The figure shows three views and two pictorial views of one solid part (mm, origin at its lowest corner). Answer the questions. Round coordinates to 2 decimals unless told otherwise and drop trailing zeros. Order: outer loops, then holes, each group sorted by start corner. A loop starts at its lowest first (then second) coordinate and runs counter-clockwise, first axis right, second up. Notation, with made-up numbers: (68.5, 39.25) - (116.5, 39.25) arc R32 cw to (116.5, 71.25) - close; hole circle Ø7 at (31.25, -17). An arc over 180 degrees is marked (long way). Answer as a JSON object with one key per item and string values. Group by question number.
Q1. A cutting plane is placed at A-A on x = 58.5. Determine the outline of the cut face in (y, z).
Q2. Consider line 1 (Z direction, x = 58.5, y = 3.1); line 2 (Z direction, x = 8, y = 2.4); line 3 (X direction, y = 4.3, z = 69) (1 decimal). Determine where each line is inside the solid, lowest interval first.
Q3. A cutting plane is placed at D-D on z = 24. Determine the outline of the cut face in (x, y), and give its area (3 significant figures).
Q4. A cutting plane is placed at C-C on y = 0.75. Count the separate pieces of the cut face and the enclosed holes in it, and give its area (3 significant figures).
Q5. A cutting plane is placed at B-B on z = 7.5. Determine the outline of the cut face in (x, y).
Q6. Given pin 1 Ø5.5 at (x, z) = (9.99, 69.75) entering from +Y; pin 2 Ø4.5 at (x, z) = (9.99, 29.75) entering from -Y (1 decimal); pin 3 Ø1 at (y, z) = (1.5, 74.5) entering from +X, each flat-ended and moving along its own axis, determine where each tip first touches the part or whether it passes through.
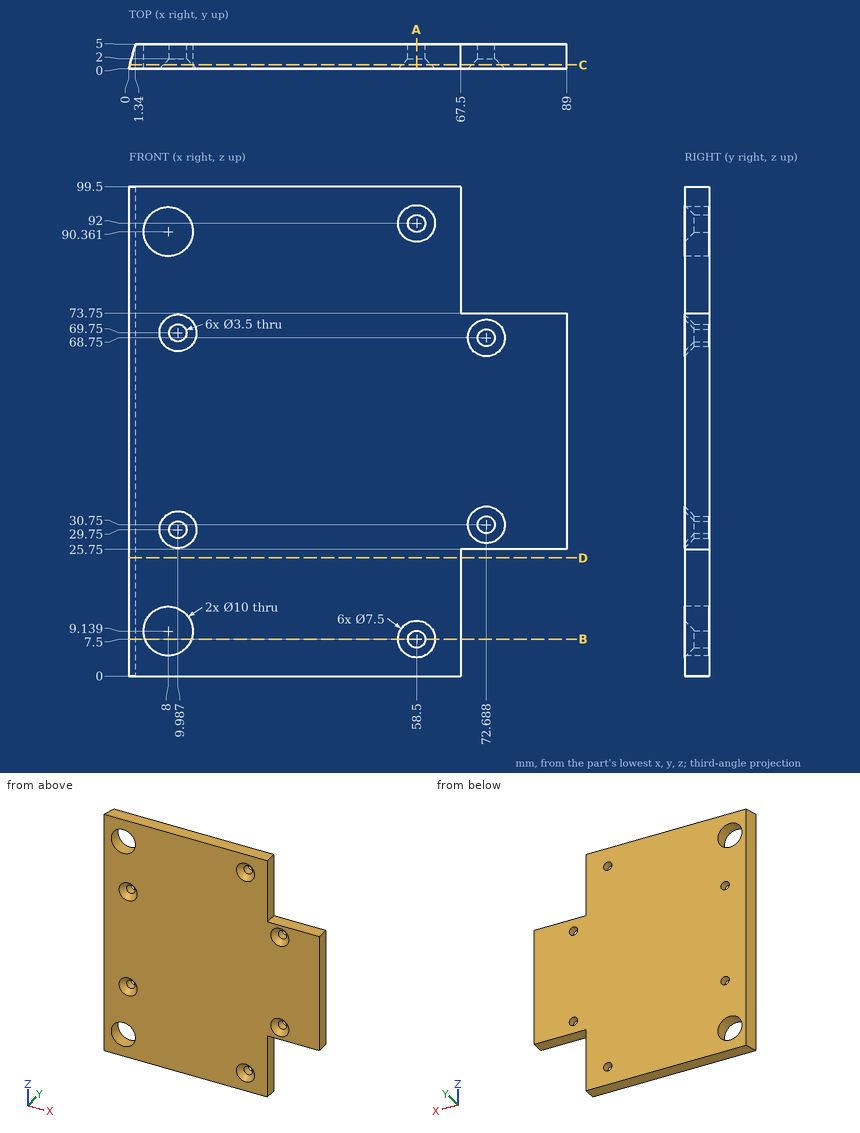
Result set:
{
 "1": {"outline": "(0, 0) - (5, 0) - (5, 5.75) - (2, 5.75) - (0, 3.75) - close; (0, 11.25) - (2, 9.25) - (5, 9.25) - (5, 90.25) - (2, 90.25) - (0, 88.25) - close; (0, 95.75) - (2, 93.75) - (5, 93.75) - (5, 99.5) - (0, 99.5) - close"},
 "2": {"line 1": "z = 0 to 5.75, 9.25 to 90.25, 93.75 to 99.5", "line 2": "z = 0 to 4.14, 14.14 to 85.36, 95.36 to 99.5", "line 3": "x = 1.2 to 8.4, 11.6 to 71, 74.4 to 89"},
 "3": {"outline": "(0, 0) - (67.5, 0) - (67.5, 5) - (1.34, 5) - close", "area": "334 mm²"},
 "4": {"separate pieces": "1", "enclosed holes": "8", "area": "7,400 mm²"},
 "5": {"outline": "(0, 0) - (3.28, 0) - (3.28, 5) - (1.34, 5) - close; (12.72, 0) - (54.75, 0) - (56.75, 2) - (56.75, 5) - (12.72, 5) - close; (60.25, 2) - (62.25, 0) - (67.5, 0) - (67.5, 5) - (60.25, 5) - close"},
 "6": {"pin 1": "stops at y = 5", "pin 2": "stops at y = 1.5", "pin 3": "stops at x = 67.5"}
}
